from build123d import *

# Parameters (mm, degrees)
SKETCH_1_R          = 5.5
SKETCH_1_R_2        = 4
EXTRUDE_1_DEPTH     = 21.5
SKETCH_2_W          = 14
SKETCH_2_H          = 3
EXTRUDE_2_DEPTH     = 23.5
SKETCH_3_R          = 3.25
CUT_EXTRUDE_1_DEPTH = 10


with BuildPart() as part:
    # 草图1 → 凸台-拉伸1 (new body)
    with BuildSketch(Plane.XY):
        Circle(SKETCH_1_R)
        Circle(SKETCH_1_R_2, mode=Mode.SUBTRACT)
    extrude(amount=EXTRUDE_1_DEPTH)

    # 草图2 → 凸台-拉伸2 (add)
    with BuildSketch(Plane(origin=(0, 0, 0), x_dir=(1, 0, 0), z_dir=(0, 1, 0))):
        with Locations((0, -20)):
            Rectangle(SKETCH_2_W, SKETCH_2_H)
    extrude(amount=EXTRUDE_2_DEPTH)

    # 草图3 → 切除-拉伸1 (cut)
    with BuildSketch(Plane(origin=(0, 0, 18.5), x_dir=(-1, 0, 0), z_dir=(0, 0, -1))):
        with Locations((0, 18.5)):
            Circle(SKETCH_3_R)
        with BuildLine():
            Line((-5.123475383, 2), (-7, 5))
            Line((-7, 5), (-7, 0))
            Line((-7, 0), (-5.5, 0))
            ThreePointArc((-5.5, 0), (-5.405049242, 1.017567048), (-5.123475383, 2))
        make_face()
        with BuildLine():
            Line((7, 5), (5.123475383, 2))
            ThreePointArc((5.123475383, 2), (5.405049242, 1.017567048), (5.5, 0))
            Line((5.5, 0), (7, 0))
            Line((7, 0), (7, 5))
        make_face()
    extrude(amount=-CUT_EXTRUDE_1_DEPTH, mode=Mode.SUBTRACT)


solid = part.part
Read the model definition and answer for the solid it produces. Units are mm, in the model's axes. A direction names the side the tool comes from. Coordinates: 2 decimals unless noted, no trailing zeros. Write each loop counter-clockwise with the first axis right and the second up, starting at its lowest first coordinate (ties: lowest second). Pieces come first, ordered by that corner, then holes. Notation, with made-up numbers: (29, 52.25) -> (55, 52.25) arc R23 cw to (55, 74.25) -> close; hole circle Ø2 at (67.5, 24.5). An arc over 180 degrees is marked (long way). Return JSON: item names as keys, results as strings.
(1) The part is cut by section A-A on x = 0. Give the vertices of the cut face in (y, z), then the cut area to 3 significant figures.
Answers below:
{"outline": "(-5.5, 0) -> (-4, 0) -> (-4, 21.5) -> (-5.5, 21.5) -> close; (0, 18.5) -> (4, 18.5) -> (4, 0) -> (5.5, 0) -> (5.5, 18.5) -> (15.25, 18.5) -> (15.25, 21.5) -> (0, 21.5) -> close; (21.75, 18.5) -> (23.5, 18.5) -> (23.5, 21.5) -> (21.75, 21.5) -> close", "area": "111 mm^2"}
(2) The part is cut by section C-C on y = 18.5. Give the vertices of the cut face in (x, z).
Answers below:
{"outline": "(-7, 18.5) -> (-3.25, 18.5) -> (-3.25, 21.5) -> (-7, 21.5) -> close; (3.25, 18.5) -> (7, 18.5) -> (7, 21.5) -> (3.25, 21.5) -> close"}
(3) The part is cut by section B-B on z = 19.5. Give the vertices of the cut face in (x, y), then the cut area to 3 significant figures.
Answers below:
{"outline": "(-7, 5) -> (-5.12, 2) arc R5.5 ccw (long way) to (5.12, 2) -> (7, 5) -> (7, 23.5) -> (-7, 23.5) -> close; hole (-4, 0) arc R4 ccw to (4, 0) -> close; hole circle Ø6.5 at (0, 18.5)", "area": "306 mm^2"}
(4) The part is cut by section D-D on z = 11. Give the vertices of the cut face in (x, y), then the cut area to 3 significant figures.
Answers below:
{"outline": "circle Ø11 at (0, 0); hole circle Ø8 at (0, 0)", "area": "44.8 mm^2"}
(5) Which of the six approach directions +Z, -Z, +X, -X, +Y, -Y give full straight-line access (tool end or side, diameter ignored) to faces 4 (the cylindrical face through (-0.867, -3.905, 10.599)), 5 (the flat face through (6.05, 3.48, 19.98)), 6 (the flat face through (-6.075, 3.521, 19.979))?
Answers below:
{"face 4": "-Z", "face 5": "+Z, -Z, +X", "face 6": "+Z, -Z, -X"}
(6) For a pull along Y with two mould halves and no side action, classify faces 1 (the cylindrical face through (0.423, 21.722, 19.979)), 2 (the flat face through (-7, 14, 20)), 3 (the flat face through (0, 23.5, 20)) as pulls with the +Y half, pulls with the -Y half, needs draft (parallel to the pull), parting line crosses it, or undercut.
Answers below:
{"face 1": "undercut", "face 2": "needs draft", "face 3": "pulls with the +Y half"}
(7) Consider line 1 along Y through (x, z) = (0, 19.4); line 2 along Y through (x, z) = (0, 14). Determine where each line is inside the solid, lowest interval first. Write a range as from..to.
Answers below:
{"line 1": "-5.5..-4, 0..15.25, 21.75..23.5", "line 2": "-5.5..-4, 4..5.5"}
(8) Each of these flat-tipped pins is pushed along its axis until it touches: P1, Ø1.5, axis at x = 1, y = 11.5, coming from the -Z side; P2, Ø0.9, axis at x = -2, z = 20, coming from the -Y side; P3, Ø10, axis at y = 3.5, z = 4, coming from the -X side. Where does it stop, or does it pass through?
Answers below:
{"P1": "z = 18.5", "P2": "y = -5.28", "P3": "x = -5.5"}
